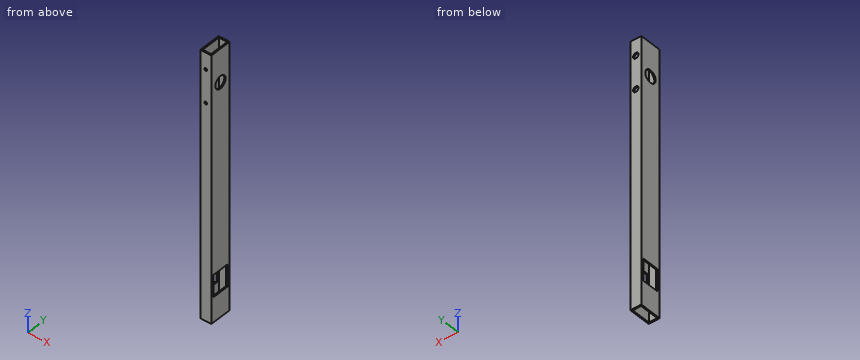
Autodesk Inventor part; units mm, degrees
ref_plane "YZ Plane" through (0, 0, 0) normal (1, 0, 0) x (0, 1, 0)
ref_plane "XZ Plane" through (0, 0, 0) normal (0, 1, 0) x (-1, 0, 0)
ref_plane "XY Plane" through (0, 0, 0) normal (0, 0, 1) x (1, 0, 0)
sketch "Sketch1" plane through (0, 0, 0) normal (0, 0, 1) x (1, 0, 0)
  line L0 (0, 0) -> (25.4, 0)
  line L1 (25.4, 0) -> (25.4, 50.8)
  line L2 (25.4, 50.8) -> (0, 50.8)
  line L3 (0, 50.8) -> (0, 0)
  line L4 (3.175, 3.175) -> (22.225, 3.175)
  line L5 (22.225, 3.175) -> (22.225, 47.625)
  line L6 (22.225, 47.625) -> (3.175, 47.625)
  line L7 (3.175, 47.625) -> (3.175, 3.175)
  dimension "d0" = 25.4
  dimension "d1" = 50.8
  dimension "d2" = 19.05
  dimension "d3" = 44.45
  dimension "d4" = 3.175
  dimension "d5" = 3.175
extrude "Extrusion1" add sketch "Sketch1" along normal blind 609.6
sketch "Sketch2" plane through (25.4, 0, 0) normal (1, 0, 0) x (0, 0, -1)
  line L0 (-609.6, 50.8) -> (-609.6, 0)
  line L1 (0, 0) -> (0, 50.8)
  line L2 (-57.15, 44.45) -> (-107.95, 44.45)
  line L3 (-107.95, 44.45) -> (-107.95, 6.35)
  line L4 (-107.95, 6.35) -> (-57.15, 6.35)
  line L5 (-57.15, 6.35) -> (-57.15, 44.45)
  line L6 (0, 0) -> (-609.6, 0)
  line L7 (0, 25.4) -> (0, 0)
  circle A0 centre (-533.4, 25.4) radius 14.2875
  dimension "d12" = 57.15
  dimension "d21" = 107.95
  dimension "d29" = 50.8
  dimension "d32" = 38.1
  dimension "d33" = 6.35
  dimension "d64" = 28.575
  dimension "d65" = 76.2
  dimension "d66" = 25.4
extrude "Extrusion2" cut sketch "Sketch2" against normal through all
sketch "Sketch5" plane through (0, 0, 0) normal (0, -1, 0) x (1, 0, 0)
  line L0 (25.4, 609.6) -> (0, 609.6)
  line L1 (25.4, 0) -> (25.4, 609.6)
  circle A0 centre (12.7, 571.5) radius 3.175
  circle A1 centre (12.7, 495.3) radius 3.175
  dimension "d53" = 38.1
  dimension "d54" = 76.2
  dimension "d55" = 12.7
  dimension "d56" = 12.7
  dimension "d57" = 6.35
extrude "Extrusion5" cut sketch "Sketch5" against normal through all
sketch "Sketch6" plane through (0, 50.8, 0) normal (0, 1, 0) x (1, 0, 0)
  circle A0 centre (12.7, -495.3) radius 3.175
  circle A1 centre (12.7, -571.5) radius 3.175
  circle A2 centre (12.7, -495.3) radius 6.35
  circle A3 centre (12.7, -571.5) radius 6.35
  dimension "d60" = 12.7
  dimension "d61" = 12.7
extrude "Extrusion6" cut sketch "Sketch6" against normal up to next
properties part number "FrameSideRail" material "Aluminum-6061"
Build history of the part. All positions in model axes, mm. Round coordinates to 2 decimals unless told otherwise and drop trailing zeros. Order: outer loops, then holes, each group sorted by start corner. A loop starts at its lowest first (then second) coordinate and runs counter-clockwise, first axis right, second up. Notation, with made-up numbers: M 68.25,44.5 L 88.25,44.5 A22 ccw 88.25,53.5 Z; hole C 84,-39.75 d6. An arc over 180 degrees is marked long. Use CSV: the item, a comma, the result in double quotes. Start each with the question number.
(1) Cut at B-B on y = 25.4. State how many separate pieces and enclosed holes the cut face has, then the cut area to 3 significant figures.
(2) Cut at C-C on z = 393. List the corners of the cut face in (x, y) (3 decimals), then the cut area to 3 significant figures.
(3) Cut at A-A on z = 533.4. List the corners of the cut face in (x, y) (1 decimal), then the cut area to 3 significant figures.
(4) Drill centre lines: probe 1 along Z at (x, y) = (12.7, 0.85) (3 decimals); probe 2 along Z at (x, y) = (1.75, 24); probe 3 along Y at (x, z) = (6.75, 468) (3 decimals). Where is each one in solid material? Low to high.
Findings:
1,separate pieces,"6"
1,enclosed holes,"0"
1,area,"3,370 mm^2"
2,outline,"M 0,0 L 25.4,0 L 25.4,50.8 L 0,50.8 Z; hole M 3.175,3.175 L 22.225,3.175 L 22.225,47.625 L 3.175,47.625 Z"
2,area,"444 mm^2"
3,outline,"M 0,0 L 25.4,0 L 25.4,11.1 L 22.2,11.1 L 22.2,3.2 L 3.2,3.2 L 3.2,11.1 L 0,11.1 Z; M 0,39.7 L 3.2,39.7 L 3.2,47.6 L 22.2,47.6 L 22.2,39.7 L 25.4,39.7 L 25.4,50.8 L 0,50.8 Z"
3,area,"262 mm^2"
4,probe 1,"z = 0 to 492.125, 498.475 to 568.325, 574.675 to 609.6"
4,probe 2,"z = 0 to 57.15, 107.95 to 519.18, 547.62 to 609.6"
4,probe 3,"y = 0 to 3.175, 47.625 to 50.8"
